```python
from build123d import *

# Parameters (mm, degrees)
REVOLVE_1_ANGLE     = 180
SHELL_1_T           = 0.5
SKETCH_1_OUTSIDE_W  = 328.82
SKETCH_1_OUTSIDE_H  = 328.82
CUT_EXTRUDE_1_DEPTH = 323
FILLET_1_R          = 2


with BuildPart() as part:
    # 草图2 → 旋转1 (revolve)
    with BuildSketch(Plane.XY):
        with BuildLine():
            Line((0, -125.2), (0, 125.2))
            ThreePointArc((0, 125.2), (-125.2, 0), (0, -125.2))
        make_face()
    revolve(axis=Axis((0, 151.670850912, 0), (0, -1, 0)), revolution_arc=REVOLVE_1_ANGLE)

    # 抽壳1
    shell_1_openings = [part.faces().sort_by_distance(p)[0] for p in [
        (0, 0, 0),
    ]]
    offset(amount=SHELL_1_T, openings=shell_1_openings)

    # 草图1 outside → 切除-拉伸1 (cut)
    with BuildSketch(Plane.XY):
        Rectangle(SKETCH_1_OUTSIDE_W, SKETCH_1_OUTSIDE_H)
        with BuildLine():
            Line((-45.921541828, 34.604363831), (-28.692164813, 21.621097001))
            Line((-28.692164813, 21.621097001), (-21.621097001, 28.692164813))
            Line((-21.621097001, 28.692164813), (-34.604363831, 45.921541828))
            ThreePointArc((-34.604363831, 45.921541828), (-40.658639918, 40.658639918), (-45.921541828, 34.604363831))
        make_face(mode=Mode.SUBTRACT)
    extrude(amount=-CUT_EXTRUDE_1_DEPTH, mode=Mode.SUBTRACT)

    # 圆角1
    # the kernel refuses this fillet: 2 mm, written as the material it takes off along each edge
    with BuildSketch(Plane(origin=(-21.621097001, 28.692164813, -115.588247879), x_dir=(-0.7071067811865281, -0.707106781186567, 0), z_dir=(0, 0, -1)), Plane(origin=(-28.692164813, 21.621097001, -115.588247879), x_dir=(-0.7986355100472948, 0.6018150231520455, 0), z_dir=(0, 0, -1))) as fillet_1_piece_1:
        with BuildLine():
            CenterArc((FILLET_1_R * 0.869286737816, FILLET_1_R), FILLET_1_R, 188, 82)
            Line((-FILLET_1_R * 0.120981330925, FILLET_1_R * 0.86082689904), (0, 0))
            Line((0, 0), (FILLET_1_R * 0.869286737816, 0))
        make_face()
    extrude(amount=9.214725038, mode=Mode.SUBTRACT)


solid = part.part
```
Could you check a few things on this model? Use its own coordinates, in mm. Coordinates: 2 decimals unless noted, no trailing zeros. Loops run counter-clockwise (first coordinate to the right, second up) from the corner with the lowest first, then second, coordinate; pieces in that order, holes last. Notation, with made-up numbers: M -28.75,27.5 L -19.75,27.5 A18 cw -19.75,62.5 Z; hole C -20.75,87 d9. An arc over 180 degrees is marked long. Put each result on its own line as item: value. Start each with the question number.
(1) Suppose I cut it at A-A on y = 37.75. Please give me the cut outline in (x, z).
(2) I need wall thicknesses on line 1 (Z direction, x = -26.75, y = 33); line 2 (Z direction, x = -39.5, y = 33.5). Which ranges of each line are inside material? Lowest first, please. Write a range as from..to.
(3) Will these pins go through, and if not, where does the flat tip stop? P1, Ø2, axis at y = 29, z = -116.5, coming from the -X side; P2, Ø3, axis at y = 39.5, z = -114, coming from the +X side; P3, Ø2, axis at y = 29.5, z = -114.5, coming from the -X side; P4, Ø3, axis at x = -26.5, y = 38, coming from the -Z side (1 decimal).
(4) Suppose I cut it at B-B on x = -41.75. Please give me the cut outline in (y, z), then the cut area to 3 significant figures.
Solutions:
1. outline: M -43.37,-111.78 A119.9 ccw -28.45,-116.47 L -28.45,-115.93 A119.37 cw -43.37,-111.22 Z
2. line 1: z = -118.3..-117.77
2. line 2: z = -114.53..-113.98
3. P1: stops at x = -39.26
3. P2: stops at x = -29.28
3. P3: stops at x = -40.47
3. P4: passes through
4. outline: M 31.46,-114.31 A118.56 ccw 39.54,-111.78 L 39.54,-111.22 A118.03 cw 31.46,-113.76 Z
4. area: 4.49 mm2
